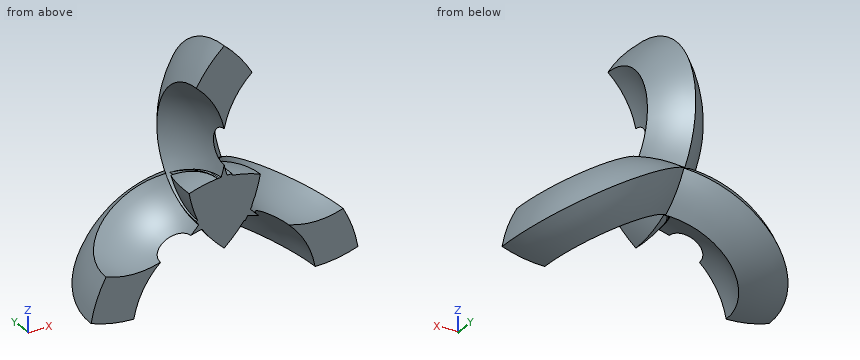
```python
from build123d import *

# Parameters (mm, degrees)
F_4_5_LEG_REVOLVE_ANGLE = 180
F_1_6_LEG_REVOLVE_ANGLE = 180
F_2_3_LEG_REVOLVE_ANGLE = 180


with BuildPart() as part:
    # Sketch4 → 4-5 leg revolve (revolve, symmetric)
    with BuildSketch(Plane.XY.offset(84.650501395)) as f_4_5_leg_revolve_sk:
        with BuildLine():
            ThreePointArc((41.52641309, 96.695760248), (14.715809322, 64.933806829), (-0.403929917, 26.216580111))
            ThreePointArc((-0.403929917, 26.216580111), (-15.523669157, 64.933806829), (-42.334272925, 96.695760248))
            ThreePointArc((-42.334272925, 96.695760248), (-23.50790032, 123.504386992), (-0.403929917, 146.728110315))
            ThreePointArc((-0.403929917, 146.728110315), (22.700040485, 123.504386992), (41.52641309, 96.695760248))
        make_face()
    revolve(axis=Axis((-124.668530377, 0, 84.650501395), (1, 0, 0)), revolution_arc=F_4_5_LEG_REVOLVE_ANGLE / 2)
    revolve(f_4_5_leg_revolve_sk.sketch, axis=Axis((-124.668530377, 0, 84.650501395), (-1, 0, 0)), revolution_arc=F_4_5_LEG_REVOLVE_ANGLE / 2)

    # Sketch5 → 1-6 leg revolve (revolve, symmetric)
    with BuildSketch(Plane(origin=(73.448953951, 0, -42.617307843), x_dir=(-0.5018671305259788, 0, -0.8649447284639755), z_dir=(0.8649447284639755, 0, -0.5018671305259788))) as f_1_6_leg_revolve_sk:
        with BuildLine():
            ThreePointArc((41.343119895, 96.695430947), (14.532414899, 64.932986617), (-0.587125541, 26.215209445))
            ThreePointArc((-0.587125541, 26.215209445), (-15.70666598, 64.932986617), (-42.517370976, 96.695430947))
            ThreePointArc((-42.517370976, 96.695430947), (-23.691050832, 123.504095778), (-0.587125541, 146.727865418))
            ThreePointArc((-0.587125541, 146.727865418), (22.516799751, 123.504095778), (41.343119895, 96.695430947))
        make_face()
    revolve(axis=Axis((136.108076543, 0, 65.372784514), (-0.5018671305259786, 0, -0.8649447284639755)), revolution_arc=F_1_6_LEG_REVOLVE_ANGLE / 2)
    revolve(f_1_6_leg_revolve_sk.sketch, axis=Axis((136.108076543, 0, 65.372784514), (0.5018671305259786, 0, 0.8649447284639755)), revolution_arc=F_1_6_LEG_REVOLVE_ANGLE / 2)

    # Sketch6 → 2-3 leg revolve (revolve, symmetric)
    with BuildSketch(Plane(origin=(-73.632148208, 0, -42.300006082), x_dir=(-0.4981305424562493, 0, 0.8671020485918846), z_dir=(-0.8671020485918844, 0, -0.49813054245624927))) as f_2_3_leg_revolve_sk:
        with BuildLine():
            ThreePointArc((41.343119895, 96.695430947), (14.532414899, 64.932986617), (-0.587125541, 26.215209445))
            ThreePointArc((-0.587125541, 26.215209445), (-15.70666598, 64.932986617), (-42.517370976, 96.695430947))
            ThreePointArc((-42.517370976, 96.695430947), (-23.691050832, 123.504095778), (-0.587125541, 146.727865418))
            ThreePointArc((-0.587125541, 146.727865418), (22.516799751, 123.504095778), (41.343119895, 96.695430947))
        make_face()
    revolve(axis=Axis((-11.439546167, 0, -150.559444204), (-0.4981305424562494, 0, 0.8671020485918846)), revolution_arc=F_2_3_LEG_REVOLVE_ANGLE / 2)
    revolve(f_2_3_leg_revolve_sk.sketch, axis=Axis((-11.439546167, 0, -150.559444204), (0.4981305424562494, 0, -0.8671020485918846)), revolution_arc=F_2_3_LEG_REVOLVE_ANGLE / 2)


solid = part.part
```
Source: CAD feature listing. Evaluate the final solid. Frame: model axes, mm. Give positions to 0.01 mm unless a question says otherwise; leave off trailing zeros. Loops run counter-clockwise (first coordinate to the right, second up) from the corner with the lowest first, then second, coordinate; pieces in that order, holes last. Notation, with made-up numbers: (-10.75, 84.25) -> (39.25, 84.25) arc R18 ccw to (39.25, 119.25) -> close; hole circle Ø11 at (-23, 65). An arc over 180 degrees is marked (long way). Use a Markdown table: item, result. Add a question column.
(1) First-contact query: pin 1 Ø1.5 at (x, z) = (122.5, -48) entering from -Y; pin 2 Ø1 at (x, z) = (114, -67) entering from +Y; pin 3 Ø6 at (y, z) = (54, 70) entering from -X. Flat tips, straight axial feed; report the tip coordinate or a pass-through.
(2) Ray query, line 1 (X direction, y = 10, z = -79); line 2 (X direction, y = 108.5, z = 46.5); line 3 (Z direction, x = -102.5, y = 86.5). Return the intervals inside material, ascending.
(3) Section query D-D (z = 8). Output: boundary loops of the cut face in (x, y).
(4) Section query C-C (x = -24). Output: boundary loops of the cut face in (y, z), then the cut area to 3 significant figures.
(5) Section query B-B (y = 91). Output: boundary loops of the cut face in (x, z), then the cut area to 3 significant figures.
(6) Section query A-A (z = -101). Output: boundary loops of the cut face in (x, y).
Checked values:
| question | item | result |
|---|---|---|
| 1 | pin 1 | y = 54.02 |
| 1 | pin 2 | y = 138.18 |
| 1 | pin 3 | x = -12.18 |
| 2 | line 1 | -189.63 to -115.88, 116.48 to 189.95 |
| 2 | line 2 | -30.23 to 29.42 |
| 2 | line 3 | -103.63 to -22.09 |
| 3 | outline | (-69.07, 92.24) arc R113.52 cw to (-40.83, 63.03) arc R176.34 ccw to (-42.33, 58.95) arc R101.26 cw to (-39.2, 54.3) arc R183.52 ccw to (-47.41, 0) -> (48.41, 0) arc R183.65 ccw to (39.61, 56.18) arc R101.26 cw to (41.53, 58.95) arc R176.34 ccw to (40.73, 61.15) arc R113.3 cw to (70.93, 92.68) arc R110.16 ccw to (13.04, 110.15) arc R176.34 ccw to (-0.4, 125.12) arc R176.34 ccw to (-14.99, 108.71) arc R108.76 ccw to start |
| 4 | outline | (0, -38.26) arc R122.91 ccw to (35.71, -32.96) arc R121.97 cw to (38.56, -33.87) arc R106.47 ccw to (43.38, -31.86) arc R126.38 cw to (90.96, -62.82) arc R156.83 ccw to (135.25, -14.46) arc R191.87 ccw to (100, 13.19) arc R122.91 ccw to (0, 207.57) -> (0, 162.08) arc R77.43 cw to (57.28, 32.56) arc R191.87 ccw to (52.83, 33.89) arc R61.28 cw to (51.78, 32.17) arc R189 ccw to (0, 39.4) -> close |
| 4 | area | 18,800 mm^2 |
| 5 | outline | (-173.14, -100.14) arc R169.38 ccw to (-80.8, -95.45) arc R88.59 cw to (-24.1, -62.88) arc R169.38 ccw to (0.6, -36.24) arc R169.38 ccw to (24.42, -61.97) arc R88.59 cw to (80.98, -94.79) arc R169.38 ccw to (173.3, -99.87) arc R169.38 ccw to (123.07, -22.25) arc R88.59 cw to (66.51, 10.57) arc R169.38 ccw to (31.31, 18.61) arc R169.38 ccw to (41.53, 51.95) arc R88.59 cw to (41.53, 117.35) arc R169.38 ccw to (-0.4, 199.75) arc R169.38 ccw to (-42.33, 117.35) arc R88.59 cw to (-42.33, 51.95) arc R169.38 ccw to (-31.69, 17.61) arc R169.38 ccw to (-65.88, 9.84) arc R88.59 cw to (-122.58, -22.74) arc R169.38 ccw to start |
| 5 | area | 36,900 mm^2 |
| 6 | outline | (-197.22, 0) -> (-128.37, 0) arc R116.93 cw to (-90.46, 86.19) arc R97.13 ccw to (-174.63, 88.78) arc R185.78 ccw to start; (91.69, 85.55) arc R117.34 cw to (128.72, 0) -> (197.42, 0) arc R186.04 ccw to (175.24, 88.09) arc R96.39 ccw to start |
